```python
from build123d import *

# Parameters (mm, degrees)
SKETCH1_R           = 4
BOSS_EXTRUDE1_DEPTH = 15
CUT_EXTRUDE1_START  = -10.1
SKETCH2_R           = 4
SKETCH2_R_2         = 3
CUT_EXTRUDE1_DEPTH  = 10.1
THREAD1_PITCH       = 1
SKETCH3_R           = 2.5
BOSS_EXTRUDE2_DEPTH = 4


with BuildPart() as part:
    # Sketch1 → Boss-Extrude1 (new body)
    with BuildSketch(Plane(origin=(0, 0, 0), x_dir=(1, 0, 0), z_dir=(0, 1, 0))):
        with Locations(Location((0, 0, 0), (0, 0, 270))):
            Circle(SKETCH1_R)
    extrude(amount=BOSS_EXTRUDE1_DEPTH)

    # Sketch2 → Cut-Extrude1 (cut)
    with BuildSketch(Plane(origin=(0, 15, 0), x_dir=(1, 0, 0), z_dir=(0, 1, 0)).offset(CUT_EXTRUDE1_START)):
        with Locations(Location((0, 0, 0), (0, 0, 270))):
            Circle(SKETCH2_R)
        with Locations(Location((0, 0, 0), (0, 0, 270))):
            Circle(SKETCH2_R_2, mode=Mode.SUBTRACT)
    extrude(amount=CUT_EXTRUDE1_DEPTH, mode=Mode.SUBTRACT)

    # Thread1: the profile of Thread Profile1 profile screwed along a right-hand helix of 6.1 turns, 8 arcs to a turn; built about Z, then put on its axis
    thread1_z = Axis((0, 0, 0), (0, 0, 1))
    thread1_corners = [(3.0003, 0, -0.000173205), (3.0003, 0, 0.875173202), (2.458734125, 0, 0.562499999), (2.458734125, 0, 0.312499999)]
    with BuildLine(mode=Mode.PRIVATE) as thread1_profile:
        Line(thread1_corners[0], thread1_corners[1])
        Line(thread1_corners[1], thread1_corners[2])
        Line(thread1_corners[2], thread1_corners[3])
        Line(thread1_corners[3], thread1_corners[0])
    thread1_cap = Face(thread1_profile.wire())
    thread1_turn_angles = [0, 22.5, 45, 67.5, 90, 112.5, 135, 157.5, 180, 202.5, 225, 247.5, 270, 292.5, 315, 337.5, 360]
    thread1_turn_weights = [1, 0.9238795325112867, 1, 0.9238795325112867, 1, 0.9238795325112867, 1, 0.9238795325112867, 1, 0.9238795325112867, 1, 0.9238795325112867, 1, 0.9238795325112867, 1, 0.9238795325112867, 1]
    thread1_turn_rails = [Edge.make_bspline([Vector(p[0], p[1], 0).rotate(thread1_z, thread1_turn_angles[k]) / thread1_turn_weights[k] + Vector(0, 0, p[2] + THREAD1_PITCH * thread1_turn_angles[k] / 360) for k in range(17)], [0, 0, 0, 1, 1, 2, 2, 3, 3, 4, 4, 5, 5, 6, 6, 7, 7, 8, 8, 8], 2, thread1_turn_weights) for p in thread1_corners]
    thread1_turn_sides = [Face.make_surface_from_curves(thread1_turn_rails[p[0]], thread1_turn_rails[p[1]]) for p in [(0, 1), (1, 2), (2, 3), (3, 0)]]
    thread1_last_angles = [2160, 2178, 2196]
    thread1_last_weights = [1, 0.9510565162951535, 1]
    thread1_last_rails = [Edge.make_bspline([Vector(p[0], p[1], 0).rotate(thread1_z, thread1_last_angles[k]) / thread1_last_weights[k] + Vector(0, 0, p[2] + THREAD1_PITCH * thread1_last_angles[k] / 360) for k in range(3)], [0, 0, 0, 1, 1, 1], 2, thread1_last_weights) for p in thread1_corners]
    thread1_last_sides = [Face.make_surface_from_curves(thread1_last_rails[p[0]], thread1_last_rails[p[1]]) for p in [(0, 1), (1, 2), (2, 3), (3, 0)]]
    thread1 = Plane(origin=(0, 15, 0), x_dir=(-1, 0, 0), z_dir=(0, -1, 0)) * Solid(Shell([*[p.moved(Location((0, 0, THREAD1_PITCH * i))) for i in range(6) for p in thread1_turn_sides], *thread1_last_sides, thread1_cap, thread1_cap.rotate(thread1_z, 2196).moved(Location((0, 0, THREAD1_PITCH * 2196 / 360)))]))
    add(thread1, mode=Mode.SUBTRACT)

    # Sketch3 → Boss-Extrude2 (add)
    with BuildSketch(Plane.XZ):
        with Locations(Location((0, 0, 0), (0, 0, 270))):
            Circle(SKETCH3_R)
    extrude(amount=BOSS_EXTRUDE2_DEPTH)


solid = part.part
```
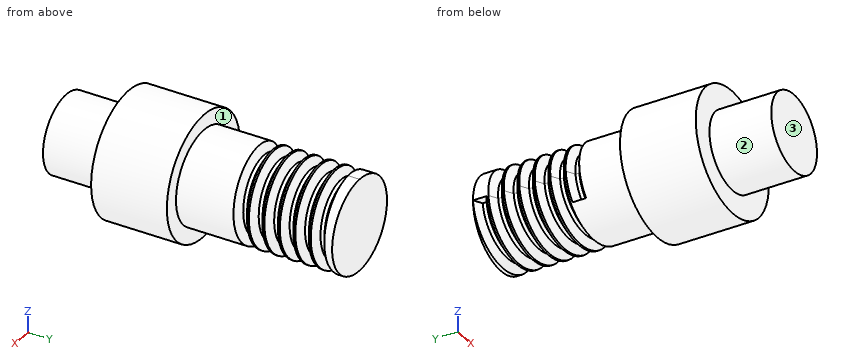
Design review of the part built by this model. Coordinates are the model's own, in mm. Face numbers are marked on the shaded views. A direction names the side the tool comes from. Give positions to 0.01 mm unless a question says otherwise; leave off trailing zeros. Order: outer loops, then holes, each group sorted by start corner. A loop starts at its lowest first (then second) coordinate and runs counter-clockwise, first axis right, second up. Notation, with made-up numbers: (9, 3.25) - (63, 3.25) arc R21 ccw to (63, 8.25) - close; hole circle Ø1 at (66, 30). An arc over 180 degrees is marked (long way). Use a Markdown table: item, result. Add a question column.
(1) Machinability: for the marked faces 1, 2 and 3, which of the approach directions +Z, -Z, +X, -X, +Y, -Y give a long, thin tool a straight path to every point of the face, cutting with its end or side? Answer none if there is none.
(2) Clearance check with a flat-ended pin moving along its axis: P1, Ø1.5, axis at y = 4, z = -2, coming from the +X side. State where the tip first meets the part, or that it passes through.
(3) Add section C-C on y = 1.5. Give the boundary of the cut face in (x, z).
(4) Add section A-A on y = 6. Give the boundary of the cut face in (x, z).
(5) Wall thickness on probe 1 along Y at (x, z) = (-3, -0.75); probe 2 along Z at (x, y) = (-1.5, 13); probe 3 along X at (y, z) = (4, -2.5): over which ranges is each line inside the solid? List them lowest first. Write a range as [from, to].
(6) Add section B-B on x = 3.5. Give the boundary of the cut face in (y, z), then the cut area to 3 significant figures.
Report:
| question | item | result |
|---|---|---|
| 1 | face 1 | +Y |
| 1 | face 2 | -Y |
| 1 | face 3 | +Z, -Z, +X, -X, -Y |
| 2 | P1 | stops at x = 3.8 |
| 3 | outline | circle Ø8 at (0, 0) |
| 4 | outline | circle Ø6 at (0, 0) |
| 5 | probe 1 | y = [0, 4.9] |
| 5 | probe 2 | z = [-2.52, 2.28] |
| 5 | probe 3 | x = [-3.12, 3.12] |
| 6 | outline | (0, -1.94) - (4.9, -1.94) - (4.9, 1.94) - (0, 1.94) - close |
| 6 | area | 19.0 mm² |
